Check sheet for the modelled part. Datum: model origin and axes. Units: mm. Face numbers are marked on the shaded views. A direction names the side the tool comes from. Coordinates: 2 decimals unless noted, no trailing zeros. Order: outer loops, then holes, each group sorted by start corner. A loop starts at its lowest first (then second) coordinate and runs counter-clockwise, first axis right, second up.
1. Thickness scan on line 1 (Y direction, x = 14.45, z = 0.7); line 2 (X direction, y = 2.75, z = 0.25); line 3 (X direction, y = -2.5, z = -5). Record the ranges inside material, lowest first.
2. Gauge pin test, flat ends, axial feed: pin 1 Ø5 at (y, z) = (-4, -0.5) entering from -X; pin 2 Ø1.6 at (x, y) = (6.45, 0) entering from -Z; pin 3 Ø1.4 at (x, y) = (12.45, 0) entering from +Z. Record the tip position at first contact, or that the pin passes through.
3. Cross-section at B-B (z = 1.25). Enter the section's corners in (x, y).
4. Cross-section at A-A (y = -2.75). Count the separate pieces of the cut face and the enclosed holes in it, then the cut area to 3 significant figures.
5. Set-up check for the marked faces 1 and 2: record each of +Z, -Z, +X, -X, +Y, -Y from which the full face is reachable in a straight line by a thin tool's end or side.
6. Cross-section at C-C (z = -3.5). Enter the section's corners in (x, y), then the cut area to 3 significant figures.
7. Draft check along Y on the marked faces 3, 4 and 5. Enter one of: released by +Y, released by -Y, zero draft, split by the parting line, or undercut.
```python
from build123d import *

# Parameters (mm, degrees)
SKETCH1_R           = 5
SKETCH1_R_2         = 2.5
BOSS_EXTRUDE1_DEPTH = 5
SKETCH2_R           = 0.6
CUT_EXTRUDE1_DEPTH  = 83.990963363
CUT_EXTRUDE2_START  = -2.5
CUT_EXTRUDE2_DEPTH  = 2.5
SKETCH4_W           = 10
SKETCH4_H           = 15
BOSS_EXTRUDE2_DEPTH = 15
SKETCH5_R           = 2.5
CUT_EXTRUDE3_DEPTH  = 15
FILLET1_R           = 5


with BuildPart() as part:
    # Sketch1 → Boss-Extrude1 (new body)
    with BuildSketch(Plane.XY):
        with BuildLine():
            Line((0, 7.5), (75, 7.5))
            ThreePointArc((75, 7.5), (82.5, 0), (75, -7.5))
            Line((75, -7.5), (0, -7.5))
            ThreePointArc((0, -7.5), (-7.5, 0), (0, 7.5))
        make_face()
        Circle(SKETCH1_R, mode=Mode.SUBTRACT)
        with Locations((75, 0)):
            Circle(SKETCH1_R_2, mode=Mode.SUBTRACT)
    extrude(amount=BOSS_EXTRUDE1_DEPTH)

    # Sketch2 → Cut-Extrude1 (cut, through all)
    with BuildSketch(Plane.XY.offset(5)):
        with Locations((4.45, 0)):
            Circle(SKETCH2_R)
        with Locations((6.45, 0)):
            Circle(SKETCH2_R)
        with Locations((8.45, 0)):
            Circle(SKETCH2_R)
        with Locations((10.45, 0)):
            Circle(SKETCH2_R)
        with Locations((12.45, 0)):
            Circle(SKETCH2_R)
        with Locations((14.45, 0)):
            Circle(SKETCH2_R)
    extrude(amount=-CUT_EXTRUDE1_DEPTH, mode=Mode.SUBTRACT)

    # Sketch3 → Cut-Extrude2 (cut)
    with BuildSketch(Plane.XY.offset(5).offset(CUT_EXTRUDE2_START)):
        with BuildLine():
            Line((14.865224913, 1.956422314), (1.038062284, 4.891055785))
            ThreePointArc((1.038062284, 4.891055785), (5, 0), (1.038062284, -4.891055785))
            Line((1.038062284, -4.891055785), (14.865224913, -1.956422314))
            ThreePointArc((14.865224913, -1.956422314), (16.45, 0), (14.865224913, 1.956422314))
        make_face()
    extrude(amount=CUT_EXTRUDE2_DEPTH, mode=Mode.SUBTRACT)

    # Sketch4 → Boss-Extrude2 (add)
    with BuildSketch(Plane(origin=(0, 7.5, 0), x_dir=(1, 0, 0), z_dir=(0, 1, 0))):
        with Locations((77.5, 2.5)):
            Rectangle(SKETCH4_W, SKETCH4_H)
    extrude(amount=-BOSS_EXTRUDE2_DEPTH)

    # Sketch5 → Cut-Extrude3 (cut)
    with BuildSketch(Plane(origin=(0, 7.5, 0), x_dir=(1, 0, 0), z_dir=(0, 1, 0))):
        with Locations(Location((77.5, 2, 0), (0, 0, 270))):
            Circle(SKETCH5_R)
    extrude(amount=-CUT_EXTRUDE3_DEPTH, mode=Mode.SUBTRACT)

    # Fillet1
    fillet1_edges = [part.edges().sort_by_distance(p)[0] for p in [
        (82.5, 0, -10),
        (72.5, 0, -10),
        (72.5, 0, 0),
        (82.5, -3.75, 5),
    ]]
    fillet(fillet1_edges, radius=FILLET1_R - 0.0001)  # a hair under: the kernel refuses the full size


solid = part.part
```
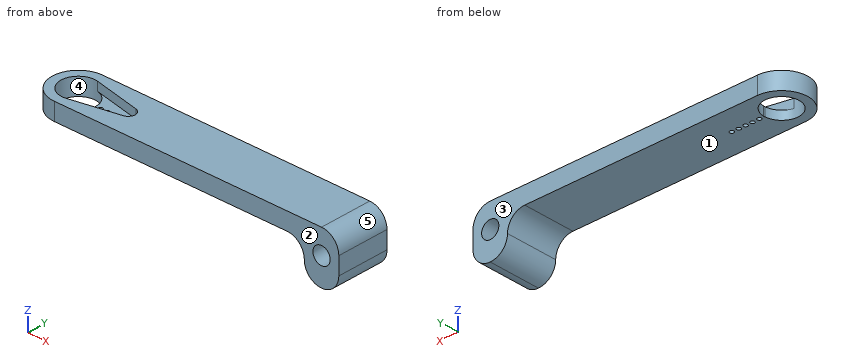
Data:
1. line 1: y = -7.5 to -0.6, 0.6 to 7.5
1. line 2: x = -6.98 to -4.18, 4.18 to 76.41, 78.59 to 82.49
1. line 3: x = 72.5 to 82.5
2. pin 1: stops at x = -7.34
2. pin 2: stops at z = 0
2. pin 3: stops at z = 2.5
3. outline: (0, -7.5) - (82.34, -7.5) - (82.34, 7.5) - (0, 7.5) arc R7.5 ccw to start; hole (4.99, -0.25) arc R0.6 ccw to (4.99, 0.25) arc R5 ccw (long way) to start; hole circle Ø1.2 at (6.45, 0); hole circle Ø1.2 at (8.45, 0); hole circle Ø1.2 at (10.45, 0); hole circle Ø1.2 at (12.45, 0); hole circle Ø1.2 at (14.45, 0)
4. separate pieces: 2
4. enclosed holes: 1
4. area: 458 mm2
5. face 1: -Z, -X, +Y, -Y
5. face 2: +Z, -Z, +X, -X, -Y
6. outline: (72.27, -7.5) - (75.5, -7.5) - (75.5, 7.5) - (72.27, 7.5) - close; (79.5, -7.5) - (82.5, -7.5) - (82.5, 7.5) - (79.5, 7.5) - close
6. area: 93.5 mm2
7. face 3: released by +Y
7. face 4: undercut
7. face 5: zero draft
